from build123d import *

# Parameters (mm, degrees)
F1_DEPTH = 63.5
F2_DEPTH = 25.4
F3_DEPTH = 7.9375


with BuildPart() as f1:
    # F0 (on Front) → F1 (new body, symmetric)
    with BuildSketch(Plane.XZ):
        Polygon((22.225, 9.525), (-41.275, 9.525), (-41.275, -9.525), (41.275, -9.525), (41.275, 9.525), align=None)
    extrude(amount=F1_DEPTH, both=True)

    # F0 (on Front) → F2 (join, symmetric)
    with BuildSketch(Plane.XZ):
        Polygon((60.325, 66.675), (60.325, 62.1792), (60.325, 42.8752), (60.325, 38.1), (111.125, 38.1), (111.125, 66.675), align=None)
        with BuildLine():
            ThreePointArc((57.15, 62.1792), (56.801973539, 62.1749562641), (56.4540060954, 62.1672695807))
            add(Edge.make_bspline(
                [(56.4540060954, 62.1672695807), (56.6863388741, 62.1719788985), (56.9183402764, 62.1759570041), (57.15, 62.1792)],
                knots=[111.0211671493, 111.0211671493, 111.0211671493, 111.0211671493, 111.6241255403, 111.6241255403, 111.6241255403, 111.6241255403], degree=3))
        make_face()
        Polygon((22.225, 9.525), (-41.275, 9.525), (-41.275, -9.525), (41.275, -9.525), (41.275, 9.525), align=None)
        with BuildLine():
            Line((22.225, 27.0002), (22.225, 9.525))
            Line((22.225, 9.525), (41.275, 9.525))
            Line((41.275, 9.525), (41.275, 27.0002))
            ThreePointArc((41.275, 27.0002), (45.9246798487, 38.2255201513), (57.15, 42.8752))
            Line((57.15, 42.8752), (60.325, 42.8752))
            Line((60.325, 42.8752), (60.325, 62.1792))
            Line((60.325, 62.1792), (57.15, 62.1792))
            add(Edge.make_bspline(
                [(56.4540060954, 62.1672695807), (56.6863388741, 62.1719788985), (56.9183402764, 62.1759570041), (57.15, 62.1792)],
                knots=[111.0211671493, 111.0211671493, 111.0211671493, 111.0211671493, 111.6241255403, 111.6241255403, 111.6241255403, 111.6241255403], degree=3))
            ThreePointArc((56.4540060954, 62.1672695807), (32.1950026375, 51.5376593284), (22.225, 27.0002))
        make_face()
    extrude(amount=F2_DEPTH, both=True)

    # F0 (on Front) → F3 (join, symmetric)
    with BuildSketch(Plane.XZ):
        with BuildLine():
            add(Edge.make_bspline(
                [(-41.275, 9.525), (-40.3382838468, 35.6428227529), (13.6751731786, 61.3001550814), (56.4540060954, 62.1672695807)],
                knots=[0, 0, 0, 0, 111.0211671493, 111.0211671493, 111.0211671493, 111.0211671493], degree=3))
            Line((-41.275, 9.525), (22.225, 9.525))
            Line((22.225, 9.525), (22.225, 27.0002))
            ThreePointArc((22.225, 27.0002), (32.1950026375, 51.5376593284), (56.4540060954, 62.1672695807))
        make_face()
    extrude(amount=F3_DEPTH, both=True)


solid = f1.part
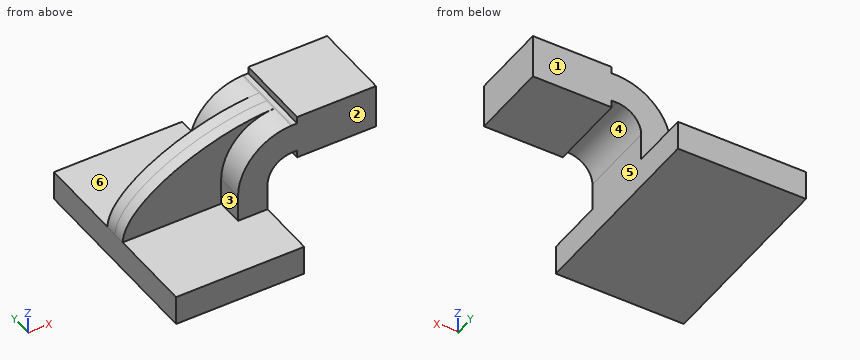
Input: part model. Units: mm. Frame: model coordinates. Face numbers are marked on the shaded views. A direction names the side the tool comes from. Coordinates: 2 decimals unless noted, no trailing zeros. Loops run counter-clockwise (first coordinate to the right, second up) from the corner with the lowest first, then second, coordinate; pieces in that order, holes last. Notation, with made-up numbers: (34, 49.5) - (92, 49.5) arc R18 cw to (92, 57.5) - close; hole circle Ø11 at (59.5, -28.5). An arc over 180 degrees is marked (long way). Answer in a Markdown table with one row per item. Add a question column.
Item 1: Section query C-C on z = -2. Return the cut outline in (x, y) (3 decimals).
Item 2: Section query B-B on x = 71. Return the cut outline in (y, z) (3 decimals), then the cut area to 3 significant figures.
Item 3: Mould query, pull axis X, two halves, no side actions, for the marked faces 4, 5 and 6. Classes: released by +X, released by -X, zero draft, split by the parting line, or undercut.
Item 4: Section query A-A on y = 22. Return the cut outline in (x, z) (3 decimals).
Item 5: Line query: line 1 along X through (y, z) = (-18, 21) (3 decimals); line 2 along X through (y, z) = (52.5, -6) (3 decimals); line 3 along Z through (x, y) = (21, -55) (3 decimals). Output: solid intervals per line, ascending. Write a range as [from, to].
Item 6: Access query for the marked faces 1, 2 and 3. Directions: +Z, -Z, +X, -X, +Y, -Y. A direction counts if a zero-diameter tool reaches every point of the face in a straight line with its end or side. Return the directions, or none.
Item 7: Contact query for flat-ended pins moving along their axis: P1, Ø5, axis at y = -2.5, z = 65, coming from the -X side (3 decimals); P2, Ø1.6, axis at x = 59, y = 10, coming from the +Z side; P3, Ø15, axis at x = 84, y = 0.5, coming from the -Z side. Output: stop coordinate, or through.
Recorded:
| question | item | result |
|---|---|---|
| 1 | outline | (-41.275, -63.5) - (41.275, -63.5) - (41.275, 63.5) - (-41.275, 63.5) - close |
| 2 | outline | (-25.4, 38.1) - (25.4, 38.1) - (25.4, 66.675) - (-25.4, 66.675) - close |
| 2 | area | 1,450 mm^2 |
| 3 | face 4 | undercut |
| 3 | face 5 | released by +X |
| 3 | face 6 | zero draft |
| 4 | outline | (-41.275, -9.525) - (41.275, -9.525) - (41.275, 27) arc R15.875 cw to (57.15, 42.875) - (60.325, 42.875) - (60.325, 38.1) - (111.125, 38.1) - (111.125, 66.675) - (60.325, 66.675) - (60.325, 62.179) - (57.15, 62.179) arc R35.18 ccw to (22.225, 27) - (22.225, 9.525) - (-41.275, 9.525) - close |
| 5 | line 1 | [22.225, 41.275] |
| 5 | line 2 | [-41.275, 41.275] |
| 5 | line 3 | [-9.525, 9.525] |
| 6 | face 1 | +Z, +X, -X, +Y |
| 6 | face 2 | +Z, +X, -X, -Y |
| 6 | face 3 | +Z, -X, -Y |
| 7 | P1 | x = 60.325 |
| 7 | P2 | z = 62.18 |
| 7 | P3 | z = 38.1 |
